Check sheet for the drawn part. Datum: minimum x, y, z corner. Units: mm. Give positions to 0.01 mm unless a question says otherwise; leave off trailing zeros. Order: outer loops, then holes, each group sorted by start corner. A loop starts at its lowest first (then second) coordinate and runs counter-clockwise, first axis right, second up. Notation, with made-up numbers: M 15,47 L 62,47 A19 cw 62,55 Z; hole C 5,-30.5 d4. An arc over 180 degrees is marked long. Answer as CSV lines item,"result". Start each with the question number.
Q1. Go/stop test with flat-tipped pins: pin 1 (2 mm diameter, centred on x = 3.28, y = 3.54, fed in from +Z); pin 2 (1.5 mm diameter, centred on x = 5.5, y = 4, fed in from -Z); pin 3 (1.5 mm diameter, centred on y = 4, z = 2.5, fed in from +X); pin 4 (3 mm diameter, centred on y = 6, z = 8.5, fed in from +X). Record where each tip stops, or that it passes through.
Q2. Section check B-B, the plane x = 2.5. Record the boundary of the cut face in (y, z) (1 decimal).
Q3. Thickness scan on line 1 (Y direction, x = 4.5, z = 7.75) (1 decimal); line 2 (X direction, y = 4.5, z = 2.5) (1 decimal); line 3 (Y direction, x = 4, z = 3) (1 decimal). Record the ranges inside material, lowest first.
Q4. Section check A-A, the plane y = 4. Record the boundary of the cut face in (x, z).
Q5. Section check D-D, the plane x = 6.25. Record the boundary of the cut face in (y, z) (1 decimal).
Q6. Mould release check, pull along Y, two halves, no side actions. Record for the marked faces 1, 2, 3 and 4: +Y half, -Y half, draft (parallel to the pull), parting line (faces both ways), or undercut.
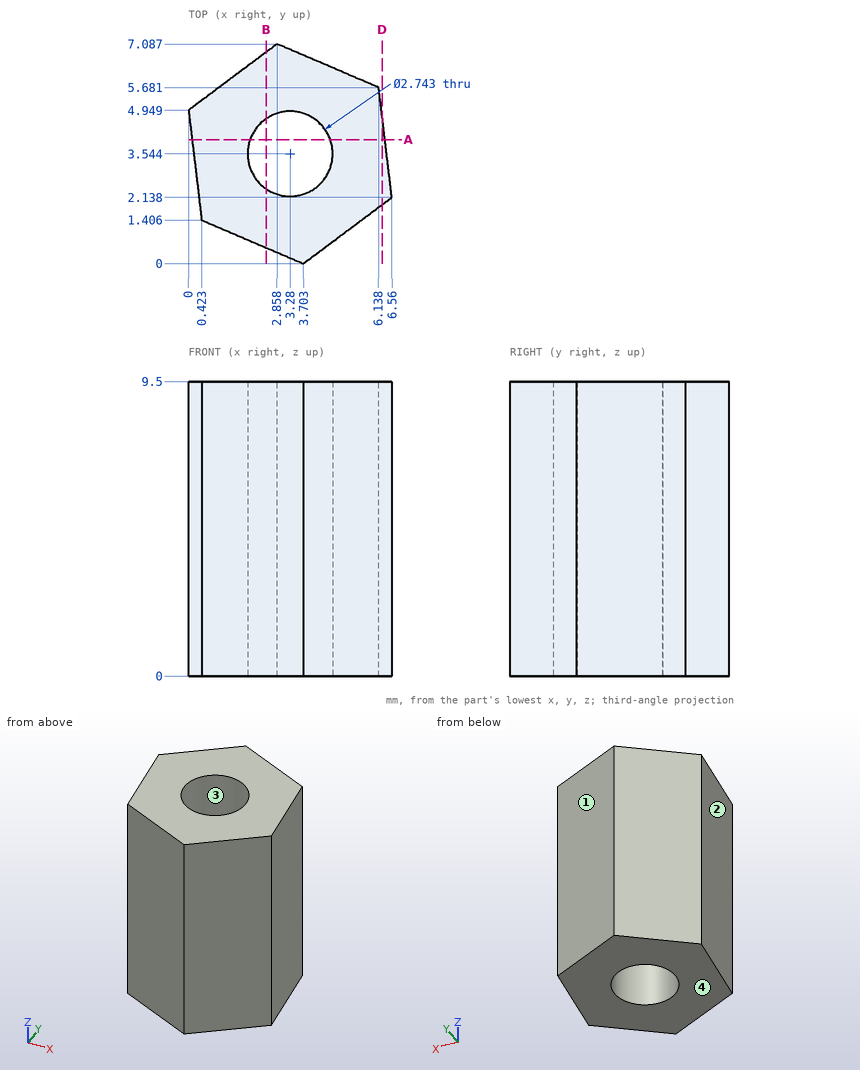
Answer block:
1,pin 1,"passes through"
1,pin 2,"stops at z = 0"
1,pin 3,"stops at x = 6.43"
1,pin 4,"stops at x = 6.28"
2,outline,"M 0.5,0 L 2.4,0 L 2.4,9.5 L 0.5,9.5 Z; M 4.7,0 L 6.8,0 L 6.8,9.5 L 4.7,9.5 Z"
3,line 1,"y = 0.6 to 2.9, 4.2 to 6.4"
3,line 2,"x = 0.1 to 2.3, 4.3 to 6.3"
3,line 3,"y = 0.2 to 2.4, 4.7 to 6.6"
4,outline,"M 0.11,0 L 1.99,0 L 1.99,9.5 L 0.11,9.5 Z; M 4.57,0 L 6.34,0 L 6.34,9.5 L 4.57,9.5 Z"
5,outline,"M 1.9,0 L 4.7,0 L 4.7,9.5 L 1.9,9.5 Z"
6,face 1,"+Y half"
6,face 2,"-Y half"
6,face 3,"undercut"
6,face 4,"draft"
